Source: CAD feature listing. Evaluate the final solid. Frame: model axes, mm. A direction names the side the tool comes from. Give positions to 0.01 mm unless a question says otherwise; leave off trailing zeros. Loops run counter-clockwise (first coordinate to the right, second up) from the corner with the lowest first, then second, coordinate; pieces in that order, holes last.
```python
from build123d import *

# Parameters (mm, degrees)
SKETCH_1_R                = 6.75
SKETCH_1_R_2              = 4.75
EXTRUDE_2_DEPTH           = 14
SKETCH_7_R                = 2.75
CUT_EXTRUDE_6_DEPTH       = 122.020659393
CUT_EXTRUDE_7_DEPTH       = 4.2
SKETCH_11_R               = 2.6
CUT_EXTRUDE_10_DEPTH      = 122.020659393
SKETCH_12_R               = 8.5
CUT_EXTRUDE_11_DEPTH      = 7
CUT_EXTRUDE_12_REACH      = 133.562
CUT_EXTRUDE_12_END_RADIUS = 8.5
FILLET_1_R                = 2.5


with BuildPart() as part:
    # Эскиз1 → Бобышка-Вытянуть2 (new body)
    with BuildSketch(Plane.XY):
        Polygon((40, 0), (40, -40), (85, -40), (85, 20), (20, 85), (-40, 85), (-40, 40), (0, 40), align=None)
        with Locations((13, 57)):
            Circle(SKETCH_1_R, mode=Mode.SUBTRACT)
        with Locations((57, 13)):
            Circle(SKETCH_1_R_2, mode=Mode.SUBTRACT)
    extrude(amount=EXTRUDE_2_DEPTH)

    # Эскиз7 → Вырез-Вытянуть6 (cut, through all)
    with BuildSketch(Plane.XY.offset(14)):
        with Locations((13, 39)):
            Circle(SKETCH_7_R)
        with Locations((13, 75)):
            Circle(SKETCH_7_R)
        with Locations((38.75, 13)):
            Circle(SKETCH_7_R)
        with Locations((75.25, 13)):
            Circle(SKETCH_7_R)
    extrude(amount=-CUT_EXTRUDE_6_DEPTH, mode=Mode.SUBTRACT)

    # Эскиз8 → Вырез-Вытянуть7 (cut)
    with BuildSketch(Plane(origin=(0, 0, 0), x_dir=(-1, 0, 0), z_dir=(0, 0, -1))):
        Polygon((-17.734272207, 75), (-15.367136104, 70.9), (-10.632863896, 70.9), (-8.265727793, 75), (-10.632863896, 79.1), (-15.367136104, 79.1), align=None)
        Polygon((-17.734272207, 39), (-15.367136104, 34.9), (-10.632863896, 34.9), (-8.265727793, 39), (-10.632863896, 43.1), (-15.367136104, 43.1), align=None)
        Polygon((-34.015727793, 13), (-36.382863896, 17.1), (-41.117136104, 17.1), (-43.484272207, 13), (-41.117136104, 8.9), (-36.382863896, 8.9), align=None)
        Polygon((-70.515727793, 13), (-72.882863896, 17.1), (-77.617136104, 17.1), (-79.984272207, 13), (-77.617136104, 8.9), (-72.882863896, 8.9), align=None)
    extrude(amount=-CUT_EXTRUDE_7_DEPTH, mode=Mode.SUBTRACT)

    # Эскиз11 → Вырез-Вытянуть10 (cut, through all)
    with BuildSketch(Plane.XY.offset(14)):
        with Locations((50, -30)):
            Circle(SKETCH_11_R)
        with Locations((75, -30)):
            Circle(SKETCH_11_R)
        with Locations((75, -10)):
            Circle(SKETCH_11_R)
        with Locations((50, -10)):
            Circle(SKETCH_11_R)
        with Locations(Location((-10, 50, 0), (0, 0, 180))):
            Circle(SKETCH_11_R)
        with Locations(Location((-30, 50, 0), (0, 0, 180))):
            Circle(SKETCH_11_R)
        with Locations(Location((-30, 75, 0), (0, 0, 180))):
            Circle(SKETCH_11_R)
        with Locations(Location((-10, 75, 0), (0, 0, 180))):
            Circle(SKETCH_11_R)
    extrude(amount=-CUT_EXTRUDE_10_DEPTH, mode=Mode.SUBTRACT)

    # Эскиз12 → Вырез-Вытянуть11 (cut)
    with BuildSketch(Plane(origin=(0, 0, 0), x_dir=(-1, 0, 0), z_dir=(0, 0, -1))):
        with Locations((-57, 13)):
            Circle(SKETCH_12_R)
    extrude(amount=-CUT_EXTRUDE_11_DEPTH, mode=Mode.SUBTRACT)

    # Вырез-Вытянуть12: up to this cylinder (the profile starts outside it)
    cut_extrude_12_end = Plane(origin=(57, 13, 1.534279), z_dir=(0, 0, -1)) * Cylinder(CUT_EXTRUDE_12_END_RADIUS, 285.124, mode=Mode.PRIVATE)
    # Эскиз13 → Вырез-Вытянуть12 (cut, up to the surface)
    with BuildSketch(Plane(origin=(52.5, 52.5, 0), x_dir=(0, 0, -1), z_dir=(0.7071067811865477, 0.7071067811865474, 0)), mode=Mode.PRIVATE) as cut_extrude_12_sk1:
        with BuildLine():
            Line((-1, -33.612698372), (0, -33.612698372))
            Line((0, -33.612698372), (0, -28.612698372))
            Line((0, -28.612698372), (-1, -28.612698372))
            ThreePointArc((-1, -28.612698372), (-3.5, -31.112698372), (-1, -33.612698372))
        make_face()
    cut_extrude_12_tool1 = extrude(cut_extrude_12_sk1.sketch, amount=-CUT_EXTRUDE_12_REACH, mode=Mode.PRIVATE) - cut_extrude_12_end
    add(cut_extrude_12_tool1.solids().sort_by_distance((74.5, 30.5, 1.534279))[0], mode=Mode.SUBTRACT)

    # Скругление1
    fillet_1_edges = [part.edges().sort_by_distance(p)[0] for p in [
        (0, 40, 7),
        (-40, 40, 7),
        (-40, 85, 7),
        (20, 85, 7),
        (85, 20, 7),
        (85, -40, 7),
        (40, -40, 7),
        (40, 0, 7),
    ]]
    fillet(fillet_1_edges, radius=FILLET_1_R)


solid = part.part
```
(1) Mould query, pull axis Y, two halves, no side actions, for faces 3 (the flat face through (16.57, 36.98, 2.07)), 4 (the flat face through (-20, 40, 7)), 5 (the flat face through (22, 37, 0)). Classes: pulls with the +Y half, pulls with the -Y half, needs draft (parallel to the pull), parting line crosses it, or undercut.
A:
face 3: undercut
face 4: pulls with the -Y half
face 5: needs draft
(2) Section D-D, the plane x = 57. Return the cut outline in (y, z), then the cut area to 3 significant figures.
A:
outline: (-40, 0) - (4.5, 0) - (4.5, 7) - (8.25, 7) - (8.25, 14) - (-40, 14) - close; (17.75, 7) - (21.5, 7) - (21.5, 0) - (48, 0) - (48, 14) - (17.75, 14) - close
area: 1,050 mm2
(3) Reachability of faces 1 (the flat face through (35.216, 10.921, 2.071)), 2 (the cylindrical face through (19.438, 59.028, 6.902)) from +Z, -Z, +X, -X, +Y, -Y: full face, straight path, thin tool, end or side. Return the list, or none.
A:
face 1: -Z
face 2: +Z, -Z
(4) Section A-A, the plane x = -10. Return the cut outline in (y, z).
A:
outline: (40, 0) - (47.4, 0) - (47.4, 14) - (40, 14) - close; (52.6, 0) - (72.4, 0) - (72.4, 14) - (52.6, 14) - close; (77.6, 0) - (85, 0) - (85, 14) - (77.6, 14) - close
(5) Section C-C, the plane z = 9. Count the separate pieces of the cut face and the enclosed holes in it, then the cut area to 3 significant figures.
A:
separate pieces: 1
enclosed holes: 14
area: 7,430 mm2
(6) First-contact query: pin 1 (5 mm diameter, centred on y = 14.5, z = 10, fed in from -X); pin 2 (1 mm diameter, centred on y = 3, z = 10, fed in from -X); pin 3 (7 mm diameter, centred on x = 38.75, y = 13, fed in from -Z). Flat tips, straight axial feed; report the tip coordinate or a pass-through.
A:
pin 1: stops at x = 23
pin 2: stops at x = 36.5
pin 3: stops at z = 4.2
(7) Section B-B, the plane y = 57. Return the cut outline in (x, z).
A:
outline: (-40, 0) - (6.25, 0) - (6.25, 14) - (-40, 14) - close; (19.75, 0) - (48, 0) - (48, 14) - (19.75, 14) - close
(8) Ray query, line 1 along Y through (x, z) = (-30, 4.5); line 2 along Y through (x, z) = (73.5, 3.75); line 3 along Y through (x, z) = (75, 11). Return the intervals inside material, ascending.
A:
line 1: y = 40 to 47.4, 52.6 to 72.4, 77.6 to 85
line 2: y = -40 to -32.12, -27.88 to -12.12, -7.88 to 8.9, 17.1 to 31.5
line 3: y = -40 to -32.6, -27.4 to -12.6, -7.4 to 10.26, 15.74 to 30
